Read the model definition and answer for the solid it produces. Units are mm, in the model's axes. A direction names the side the tool comes from. Give positions to 0.01 mm unless a question says otherwise; leave off trailing zeros. Loops run counter-clockwise (first coordinate to the right, second up) from the corner with the lowest first, then second, coordinate; pieces in that order, holes last. Notation, with made-up numbers: (6.25, 62) - (53.25, 62) arc R16 ccw to (53.25, 71) - close; hole circle Ø7 at (33.25, 45.25). An arc over 180 degrees is marked (long way). Write each question's results on one line, items separated by ' | '. Start each with the question number.
Q1. Given pin 1 (12 mm diameter, centred on y = -29.5, z = -23, fed in from -X); pin 2 (3 mm diameter, centred on y = -251.5, z = 94, fed in from -X); pin 3 (6 mm diameter, centred on x = 957, z = 139.5, fed in from -Y), each flat-ended and moving along its own axis, determine where each tip first touches the part or whether it passes through.
Q2. For faces 1 (the cylindrical face through (295.8, -14.985, -0.66)), 2 (the flat face through (630, 5, 1)), determine the directions among +Z, -Z, +X, -X, +Y, -Y from which every point of the face is accessible in a straight line to the end or side of a thin tool.
Q3. Find the intervals of material crossed by line 1 (Y direction, x = 1296.5, z = 151.5); line 2 (Z direction, x = 1279.5, y = 332); line 3 (Y direction, x = 749, z = 37), in increasing order. Write a range as from..to.
Q4. The part is cut by section B-B, the plane x = 1345. State how many separate pieces and enclosed holes the cut face has, plus the area to 3 significant figures.
Q5. Determine the mould class of faces 3 (the flat face through (614.79, 40.39, -4.58)), 4 (the flat face through (0, 0, 0)) for opening direction Z: +Z half, -Z half, draft (parallel to the pull), parting line (faces both ways), or undercut.
Q6. The part is cut by section A-A, the plane x = 408.5. Write down the section's boundary in (y, z).
Autodesk Inventor part; units mm, degrees
ref_plane "Plan de construction1" through (630, -8.3153, 57.1331) normal (-0.8660254, 0.4645044, -0.1850289) x (0, -0.3700577, -0.9290088)
ref_plane "Plan de construction2" through (630, -45.3211, -35.7678) normal (-0.8660254, -0.0720125, 0.494787) x (0, 0.989574, 0.144025)
ref_plane "Plan de construction3" through (630, 53.6363, -21.3653) normal (-0.8660254, -0.3924919, -0.3097582) x (0, -0.6195163, 0.7849838)
sketch "Esquisse2" plane through (0, 0, 0) normal (1, 0, 0) x (0, 1, 0)
  circle A0 centre (0, 0) radius 15
  dimension "d3" = 30
extrude "Extrusion1" add sketch "Esquisse2" along normal blind 600
sketch "Esquisse3" plane through (600, 0, 0) normal (1, 0, 0) x (0, 0, -1)
  circle A0 centre (0, 0) radius 15 construction
  line L0 (35.7678, -45.3211) -> (21.3653, 53.6363)
  line L1 (21.3653, 53.6363) -> (-57.1331, -8.3153)
  line L2 (-57.1331, -8.3153) -> (35.7678, -45.3211)
  line L3 (54.348, 0) -> (-75.7133, 0) construction
  dimension "d12" = 60
  dimension "d13" = 60
  dimension "d14" = 60
  dimension "d16" = 100
  dimension "d17" = 86.6025
  dimension "d18" = 28.8675
  dimension "d19" = 28.8675
  dimension "d20" = 28.8675
  dimension "d21" = 38.281
extrude "Extrusion2" add sketch "Esquisse3" along normal blind 30
ref_plane "Plan de construction1" through (630, -8.3153, 57.1331) normal (-0.8660254, 0.4645044, -0.1850289) x (0, -0.3700577, -0.9290088)
ref_plane "Plan de construction2" through (630, -45.3211, -35.7678) normal (-0.8660254, -0.0720125, 0.494787) x (0, 0.989574, 0.144025)
ref_plane "Plan de construction3" through (630, 53.6363, -21.3653) normal (-0.8660254, -0.3924919, -0.3097582) x (0, -0.6195163, 0.7849838)
sketch "Esquisse4" plane through (630, -45.3211, -35.7678) normal (-0.8660254, -0.0720125, 0.494787) x (0, 0.989574, 0.144025)
  line L0 (0, 15) -> (100, 15) construction
  line L1 (100, 15) -> (100, 0) construction
  line L2 (0, 0) -> (100, 0) construction
  line L3 (0, 15) -> (0, 0) construction
  circle A0 centre (50, 7.5) radius 10
  line L4 (50, 753.3118) -> (50, -218.5479) construction
  point P0 (50, 290)
  dimension "d25" = 20
  dimension "d26" = 15
  dimension "d27" = 7.5
extrude "Extrusion3" add sketch "Esquisse4" along normal blind 40 and the other way blind 1000
sketch "Esquisse5" plane through (630, 53.6363, -21.3653) normal (-0.8660254, -0.3924919, -0.3097582) x (0, -0.6195163, 0.7849838)
  line L0 (0, 15) -> (100, 15) construction
  line L1 (100, 15) -> (100, 0) construction
  line L2 (0, 0) -> (100, 0) construction
  line L3 (0, 15) -> (0, 0) construction
  circle A0 centre (50, 7.5) radius 10
  line L4 (50, 845.2082) -> (50, -1048.939) construction
  point P0 (50, 290)
  dimension "d32" = 20
  dimension "d33" = 7.5
extrude "Extrusion4" add sketch "Esquisse5" along normal blind 40 and the other way blind 1000
sketch "Esquisse6" plane through (630, -8.3153, 57.1331) normal (-0.8660254, 0.4645044, -0.1850289) x (0, -0.3700577, -0.9290088)
  line L0 (0, 15) -> (100, 15) construction
  line L1 (100, 15) -> (100, 0) construction
  line L2 (0, 0) -> (100, 0) construction
  line L3 (0, 15) -> (0, 0) construction
  circle A0 centre (50, 7.5) radius 10
  line L4 (50, 943.564) -> (50, -1296.7643) construction
  point P0 (50, 290)
  dimension "d38" = 20
  dimension "d39" = 7.5
extrude "Extrusion5" add sketch "Esquisse6" along normal blind 40 and the other way blind 1000
equation "\"d18\" = 0.333333 * d17"
equation "\"d19\" = 0.333333 * d17"
equation "\"d27\" = 0.5 * d26"
properties part number "P003_tripod"
Check sheet entries:
1) pin 1: stops at x = 600 | pin 2: stops at x = 1010.35 | pin 3: stops at y = 165.42
2) face 1: -X | face 2: +X
3) line 1: y = -401.8..-381.85 | line 2: z = 249.65..263.68 | line 3: y = -109.44..-87.44
4) separate pieces: 3 | enclosed holes: 0 | area: 1,090 mm^2
5) face 3: undercut | face 4: draft
6) outline: circle Ø30 at (0, 0)
